from build123d import *

# Parameters (mm, degrees)
F0_R     = 127
F0_R_2   = 31.774252
F1_DEPTH = 76.2
F3_DEPTH = 127
F5_DEPTH = 127
F6_R     = 113.822054
F6_R_2   = 38.1
F7_DEPTH = 50.8
F8_W     = 50.940839
F8_H     = 7.62
F8_W_2   = 7.62
F8_H_2   = 50.8
F9_DEPTH = 76.2


with BuildPart() as f1:
    # F0 (on Front) → F1 (new body)
    with BuildSketch(Plane.XZ):
        Circle(F0_R)
        Circle(F0_R_2, mode=Mode.SUBTRACT)
    extrude(amount=F1_DEPTH)

    # F2 (on Right) → F3 (cut, symmetric)
    with BuildSketch(Plane.YZ):
        Polygon((-63.5, 12.7), (-76.2, 12.7), (-76.2, -12.7), (-63.5, -12.7), (-63.5, -9.525), (-58.42, -9.525), (-58.42, -12.7), (-55.245, -12.7), (-55.245, 12.7), (-58.42, 12.7), (-58.42, 9.525), (-63.5, 9.525), align=None)
    extrude(amount=F3_DEPTH, both=True, mode=Mode.SUBTRACT)

    # F4 (on Top) → F5 (cut, symmetric)
    with BuildSketch(Plane.XY):
        Polygon((12.7, -76.2), (12.7, -63.5), (9.525, -63.5), (9.524411, -58.42), (12.728042, -58.42), (12.728042, -55.245), (-12.7, -55.245), (-12.7, -58.42), (-9.52559, -58.42), (-9.525, -63.5), (-12.7, -63.5), (-12.7, -76.2), align=None)
    extrude(amount=F5_DEPTH, both=True, mode=Mode.SUBTRACT)

    # F6 (on face) → F7 (cut)
    with BuildSketch(Plane(origin=(0, 0, 0), x_dir=(-1, 0, 0), z_dir=(0, 1, 0))):
        Circle(F6_R)
        Circle(F6_R_2, mode=Mode.SUBTRACT)
    extrude(amount=-F7_DEPTH, mode=Mode.SUBTRACT)

    # F8 (on Front) → F9 (cut)
    with BuildSketch(Plane.XZ):
        with Locations((76.30205, 0)):
            Rectangle(F8_W, F8_H)
        with Locations((-76.30205, 0)):
            Rectangle(F8_W, F8_H)
        with Locations((0, -76.2)):
            Rectangle(F8_W_2, F8_H_2)
        with Locations((0, 76.2)):
            Rectangle(F8_W_2, F8_H_2)
    extrude(amount=F9_DEPTH, mode=Mode.SUBTRACT)


solid = f1.part
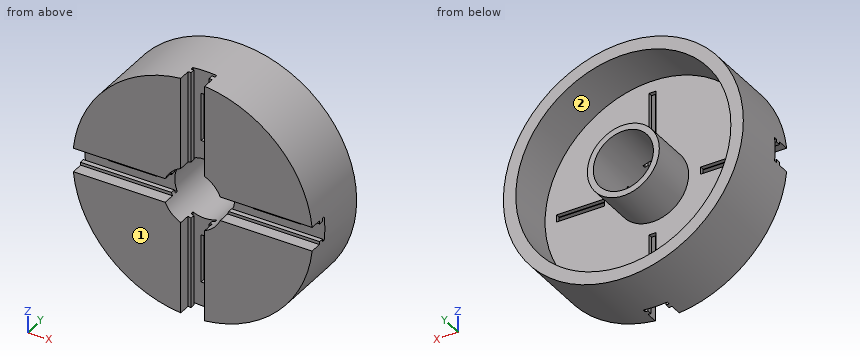
The model under review builds one solid part; all positions refer to its coordinate system, in mm. Face numbers are marked on the shaded views. A direction names the side the tool comes from. Round coordinates to 2 decimals unless told otherwise and drop trailing zeros. Write each loop counter-clockwise with the first axis right and the second up, starting at its lowest first coordinate (ties: lowest second). Pieces come first, ordered by that corner, then holes. Notation, with made-up numbers: M 71.5,9.5 L 82.5,9.5 A25 ccw 82.5,45.5 Z; hole C 15,9.5 d2. An arc over 180 degrees is marked long. Use a Markdown table: item, result. Add a question column.
Q1. Insertion check: pin 1 (8 mm diameter, centred on y = -66, z = -88.5, fed in from +X); pin 2 (3.5 mm diameter, centred on y = -53, z = 75.5, fed in from +X); pin 3 (10 mm diameter, centred on x = 89.5, y = -70, fed in from +Z). Each pin has a flat end and moves straight along its axis. Give the tip position at first contact, or say it passes through.
Q2. Machinability: for the marked faces 1 and 2, which of the approach directions +Z, -Z, +X, -X, +Y, -Y give a long, thin tool a straight path to every point of the face, cutting with its end or side? Answer none if there is none.
Q3. To check wall thickness, follow line 1 (Z direction, x = 0, y = -38); line 2 (Z direction, x = -15.5, y = -56.5); line 3 (X direction, y = -53, z = 6). State the ranges of each line that lie inside material, in increasing order.
Q4. We need section D-D, the plane y = -42.5. State the section outline as (x, z) points, plus the area to 3 significant figures.
Q5. We need section C-C, the plane z = 87. State the section outline as (x, y) points (1 decimal), plus the area to 3 significant figures.
Q6. We need section A-A, the plane x = 0. State the section outline as (y, z) points (3 decimals).
Q7. We need section B-B, the plane z = 0. State the section outline as (x, y) points (3 decimals), plus the area to 3 significant figures.
Findings below:
| question | item | result |
|---|---|---|
| 1 | pin 1 | stops at x = 94.81 |
| 1 | pin 2 | stops at x = 103.39 |
| 1 | pin 3 | stops at z = 94.81 |
| 2 | face 1 | +Z, -Z, +X, -X, -Y |
| 2 | face 2 | +Y |
| 3 | line 1 | z = -127 to -113.82, -38.1 to -31.77, 31.77 to 38.1, 113.82 to 127 |
| 3 | line 2 | z = -126.05 to -27.74, 27.74 to 126.05 |
| 3 | line 3 | x = -126.86 to -31.2, 31.2 to 126.86 |
| 4 | outline | C 0,0 d254; C 0,0 d76.2; hole C 0,0 d227.64; hole C 0,0 d63.55 |
| 4 | area | 11,400 mm² |
| 5 | outline | M -92.5,-76.2 L -12.7,-76.2 L -12.7,-63.5 L -9.5,-63.5 L -9.5,-58.4 L -12.7,-58.4 L -12.7,-55.2 L -3.8,-55.2 L -3.8,-50.8 L -73.4,-50.8 L -73.4,0 L -92.5,0 Z; M 3.8,-55.2 L 12.7,-55.2 L 12.7,-58.4 L 9.5,-58.4 L 9.5,-63.5 L 12.7,-63.5 L 12.7,-76.2 L 92.5,-76.2 L 92.5,0 L 73.4,0 L 73.4,-50.8 L 3.8,-50.8 Z |
| 5 | area | 6,110 mm² |
| 6 | outline | M -55.245,-127 L 0,-127 L 0,-113.822 L -50.8,-113.822 L -50.8,-101.6 L -55.245,-101.6 Z; M -55.245,-50.8 L -50.8,-50.8 L -50.8,-38.1 L 0,-38.1 L 0,-31.774 L -55.245,-31.774 Z; M -55.245,31.774 L 0,31.774 L 0,38.1 L -50.8,38.1 L -50.8,50.8 L -55.245,50.8 Z; M -55.245,101.6 L -50.8,101.6 L -50.8,113.822 L 0,113.822 L 0,127 L -55.245,127 Z |
| 7 | outline | M -127,-55.245 L -101.772,-55.245 L -101.772,-50.8 L -113.822,-50.8 L -113.822,0 L -127,0 Z; M -50.832,-55.245 L -31.774,-55.245 L -31.774,0 L -38.1,0 L -38.1,-50.8 L -50.832,-50.8 Z; M 31.774,-55.245 L 50.832,-55.245 L 50.832,-50.8 L 38.1,-50.8 L 38.1,0 L 31.774,0 Z; M 101.772,-55.245 L 127,-55.245 L 127,0 L 113.822,0 L 113.822,-50.8 L 101.772,-50.8 Z |
| 7 | area | 2,380 mm² |
